Check sheet for the modelled part. Datum: model origin and axes. Units: mm. A direction names the side the tool comes from. Round coordinates to 2 decimals unless told otherwise and drop trailing zeros. Loops run counter-clockwise (first coordinate to the right, second up) from the corner with the lowest first, then second, coordinate; pieces in that order, holes last. Notation, with made-up numbers: (6.25, 34.5) -> (18.25, 34.5) arc R18 ccw to (18.25, 54.5) -> close; hole circle Ø3 at (65, 64). An arc over 180 degrees is marked (long way). One line per item, written item: value. Start each with the question number.
1. Go/stop test with flat-tipped pins: pin 1 (1.8 mm diameter, centred on x = 38.5, y = 3.5, fed in from -Z); pin 2 (3 mm diameter, centred on x = 38.5, y = 2.5, fed in from +Z); pin 3 (3 mm diameter, centred on y = 4, z = 0, fed in from +X). Record where each tip stops, or that it passes through.
2. Release check for a two-part mould opening along Z. For faces 1 (the face through (-38, 3, 13)), 2 (the face through (-31, 3, -3.657)), 3 (the face through (-41, 3, -8)) record: +Z half, -Z half, draft (parallel to the pull), parting line (faces both ways), or undercut.
3. Cross-section at B-B on z = -0.5. Record the cut outline in (x, y).
4. Material ranges on L1, parallel to Z at x = 29, y = 4.2; L2, parallel to X at y = 4.15, z = 6; L3, parallel to X at y = 4.3, z = 2.5, recorded low to high.
5. Cross-section at C-C on z = -17. Record the cut outline in (x, y).
6. Set-up check for faces 4 (the face through (35, 3, 17)), 5 (the face through (-35, 3, 16)), 6 (the face through (28, 3, 2.157)), 7 (the face through (-33, 3, -3)), 8 (the face through (-28, 3, -2.157)): record each of +Z, -Z, +X, -X, +Y, -Y from which the full face is reachable in a straight line by a thin tool's end or side.
7. Cross-section at A-A on z = 11. Record the cut outline in (x, y).
from build123d import *

# Parameters (mm, degrees)
SKETCH1_W           = 6
SKETCH1_H           = 25
BOSS_EXTRUDE1_DEPTH = 6


with BuildPart() as part:
    # Sketch1 → Boss-Extrude1 (new body)
    with BuildSketch(Plane(origin=(0, 0, 0), x_dir=(1, 0, 0), z_dir=(0, 1, 0))):
        Polygon((35, 20), (-35, 20), (-35, 13), (-41, 13), (-41, 2.156563888), (-33, 2.156563888), (-33, 3.656563888), (-29.8, 3.656563888), (-29.8, 2.156563888), (-25.8, 2.156563888), (-25.8, 1.843436112), (-25.8, -1.843436112), (-25.8, -2.156563888), (-29.8, -2.156563888), (-29.8, -3.656563888), (-33, -3.656563888), (-33, -2.156563888), (-41, -2.156563888), (-41, -13), (-35, -13), (-35, -20), (35, -20), (35, -13), (41, -13), (41, -2.156563888), (33, -2.156563888), (33, -3.656563888), (29.8, -3.656563888), (29.8, -2.156563888), (25.8, -2.156563888), (25.8, -1.843436112), (25.8, 1.843436112), (25.8, 2.156563888), (29.8, 2.156563888), (29.8, 3.656563888), (33, 3.656563888), (33, 2.156563888), (41, 2.156563888), (41, 13), (35, 13), align=None)
        with Locations((-18, 0)):
            Rectangle(SKETCH1_W, SKETCH1_H, mode=Mode.SUBTRACT)
    extrude(amount=BOSS_EXTRUDE1_DEPTH)


solid = part.part
Taken from the geometry:
1. pin 1: stops at z = -13
1. pin 2: stops at z = 13
1. pin 3: stops at x = 25.8
2. face 1: +Z half
2. face 2: undercut
2. face 3: draft
3. outline: (-25.8, 0) -> (-21, 0) -> (-21, 6) -> (-25.8, 6) -> close; (-15, 0) -> (25.8, 0) -> (25.8, 6) -> (-15, 6) -> close
4. L1: z = -20 to -2.16, 2.16 to 20
4. L2: x = -41 to -21, -15 to 41
4. L3: x = -41 to -33, -29.8 to -21, -15 to 29.8, 33 to 41
5. outline: (-35, 0) -> (35, 0) -> (35, 6) -> (-35, 6) -> close
6. face 4: +Z, +X, +Y, -Y
6. face 5: +Z, -X, +Y, -Y
6. face 6: +X, +Y, -Y
6. face 7: +Y, -Y
6. face 8: -X, +Y, -Y
7. outline: (-41, 0) -> (-21, 0) -> (-21, 6) -> (-41, 6) -> close; (-15, 0) -> (41, 0) -> (41, 6) -> (-15, 6) -> close
